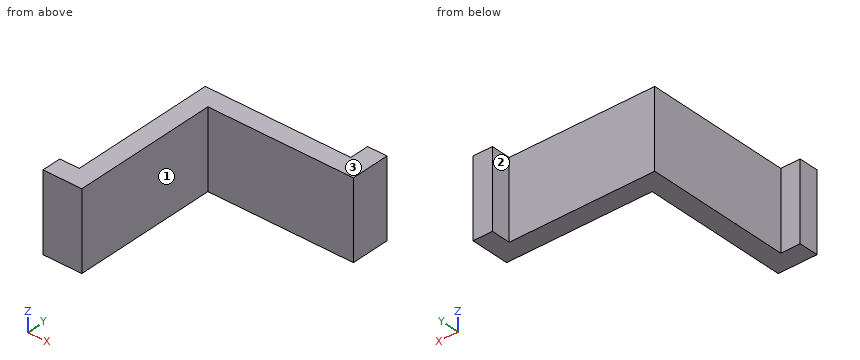
```python
from build123d import *

# Parameters (mm, degrees)
F1_DEPTH = 25.4
F3_W     = 6.35
F3_H     = 25.4
F4_DEPTH = 6.35
F2_W     = 6.35
F2_H     = 25.4
F5_DEPTH = 6.35


with BuildPart() as f1:
    # F0 (on Top) → F1 (new body)
    with BuildSketch(Plane.XY):
        Polygon((-31.75, -22.225), (-25.4, -22.225), (-25.4, 25.4), (22.225, 25.4), (22.225, 31.75), (-31.75, 31.75), align=None)
    extrude(amount=F1_DEPTH)

    # F3 (on face) → F4 (join)
    with BuildSketch(Plane(origin=(0, 31.75, 0), x_dir=(-1, 0, 0), z_dir=(0, 1, 0))):
        with Locations((-19.05, 12.7)):
            Rectangle(F3_W, F3_H)
    extrude(amount=F4_DEPTH)

    # F2 (on face) → F5 (join)
    with BuildSketch(Plane(origin=(-31.75, 0, 0), x_dir=(0, -1, 0), z_dir=(-1, 0, 0))):
        with Locations((19.05, 12.7)):
            Rectangle(F2_W, F2_H)
    extrude(amount=F5_DEPTH)


solid = f1.part
```
Work out the finished part from the listing and answer in its coordinate system (mm). Face numbers are marked on the shaded views. A direction names the side the tool comes from. Coordinates: 2 decimals unless noted, no trailing zeros. Write each loop counter-clockwise with the first axis right and the second up, starting at its lowest first coordinate (ties: lowest second). Pieces come first, ordered by that corner, then holes.
Q1. A cutting plane is placed at A-A, the plane z = 6.5. Give the vertices of the cut face in (x, y) (3 decimals), then the cut area to 3 significant figures.
Q2. A cutting plane is placed at C-C, the plane x = 4. Give the vertices of the cut face in (y, z), then the cut area to 3 significant figures.
Q3. Which of the six approach directions +Z, -Z, +X, -X, +Y, -Y give full straight-line access (tool end or side, diameter ignored) to the marked faces 1, 2 and 3?
Q4. Each of these flat-tipped pins is pushed along its axis until it touches: pin 1 Ø6 at (y, z) = (10, 19) entering from -X; pin 2 Ø5 at (x, z) = (-36, 10) entering from +Y (3 decimals); pin 3 Ø7.5 at (y, z) = (-4, 16.5) entering from +X. Where does it stop, or does it pass through?
Q5. A cutting plane is placed at B-B, the plane y = -12. Give the vertices of the cut face in (x, z).
Q6. Find the intervals of material crossed by line 1 (X direction, y = -16, z = 23.25); line 2 (Y direction, x = -25, z = 22.5); line 3 (X direction, y = 30, z = 3) (3 decimals), in increasing order.
Findings below:
1. outline: (-38.1, -22.225) - (-25.4, -22.225) - (-25.4, 25.4) - (22.225, 25.4) - (22.225, 38.1) - (15.875, 38.1) - (15.875, 31.75) - (-31.75, 31.75) - (-31.75, -15.875) - (-38.1, -15.875) - close
1. area: 726 mm2
2. outline: (25.4, 0) - (31.75, 0) - (31.75, 25.4) - (25.4, 25.4) - close
2. area: 161 mm2
3. face 1: +Z, -Z, +X, -Y
3. face 2: +Z, -Z, -X, +Y
3. face 3: +Z, +X, -X, +Y, -Y
4. pin 1: stops at x = -31.75
4. pin 2: stops at y = -15.875
4. pin 3: stops at x = -25.4
5. outline: (-31.75, 0) - (-25.4, 0) - (-25.4, 25.4) - (-31.75, 25.4) - close
6. line 1: x = -38.1 to -25.4
6. line 2: y = 25.4 to 31.75
6. line 3: x = -31.75 to 22.225
